Could you check a few things on this model? Use its own coordinates, in mm. Coordinates: 2 decimals unless noted, no trailing zeros. Order: outer loops, then holes, each group sorted by start corner. A loop starts at its lowest first (then second) coordinate and runs counter-clockwise, first axis right, second up. Notation, with made-up numbers: (28, 79) - (45, 79) arc R16 cw to (45, 89) - close; hole circle Ø11 at (-38, 74.25). An arc over 180 degrees is marked (long way). One line per item, written item: value.
from build123d import *

# Parameters (mm, degrees)
SKETCH1_W           = 145
SKETCH1_H           = 145
BOSS_EXTRUDE1_DEPTH = 3
FILLET1_R           = 2.5
SKETCH2_W           = 25
SKETCH2_H           = 15
CUT_EXTRUDE1_DEPTH  = 1


with BuildPart() as part:
    # Sketch1 → Boss-Extrude1 (new body)
    with BuildSketch(Plane(origin=(0, 0, 0), x_dir=(1, 0, 0), z_dir=(0, 1, 0))):
        with Locations((72.5, 72.5)):
            Rectangle(SKETCH1_W, SKETCH1_H)
    extrude(amount=BOSS_EXTRUDE1_DEPTH)

    # Fillet1
    fillet1_edges = [part.edges().sort_by_distance(p)[0] for p in [
        (145, 3, -72.5),
        (72.5, 3, -145),
        (0, 3, -72.5),
        (72.5, 3, 0),
    ]]
    fillet(fillet1_edges, radius=FILLET1_R)

    # Sketch2 → Cut-Extrude1 (cut)
    with BuildSketch(Plane.XZ):
        with Locations((72.5, -37.5)):
            Rectangle(SKETCH2_W, SKETCH2_H)
    extrude(amount=-CUT_EXTRUDE1_DEPTH, mode=Mode.SUBTRACT)


solid = part.part
Item 1: Thinking about a two-plate mould opening in X: for faces 1 (the face through (72, 1, -37)), 2 (the face through (72, 3, -73)), which applies, pulls with the +X half, pulls with the -X half, needs draft (parallel to the pull), parting line crosses it, or undercut?
Conclusion:
face 1: undercut
face 2: needs draft
Item 2: If I drill on probe 1 along X at (y, z) = (0.65, -40); probe 2 along X at (y, z) = (0.85, -46.5); probe 3 along X at (y, z) = (2.8, -128), over which ranges is the centre line in solid material (lowest first)?
Conclusion:
probe 1: 0 to 60, 85 to 145
probe 2: 0.02 to 144.98
probe 3: 1.52 to 143.48
Item 3: I want a section at B-B on x = 64.5. Please give me the cut outline in (y, z).
Conclusion:
outline: (0, -145) - (0.5, -145) arc R2.5 ccw to (3, -142.5) - (3, -2.5) arc R2.5 ccw to (0.5, 0) - (0, 0) - (0, -30) - (1, -30) - (1, -45) - (0, -45) - close
Item 4: I want a section at A-A on z = -32.5. Please give me the cut outline in (x, y).
Conclusion:
outline: (0, 0) - (60, 0) - (60, 1) - (85, 1) - (85, 0) - (145, 0) - (145, 0.5) arc R2.5 ccw to (142.5, 3) - (2.5, 3) arc R2.5 ccw to (0, 0.5) - close
Item 5: I'm going to push flat-ended pins straight in: pin 1 Ø4.5 at (x, z) = (73.5, -37) entering from -Y; pin 2 Ø1.5 at (y, z) = (1.5, -118) entering from -X. Where does each tip first touch, or does it pass through?
Conclusion:
pin 1: y = 1
pin 2: x = 0.01
